The listing builds one solid part. Answer for the finished solid, in the listing's coordinates (mm). A direction names the side the tool comes from. Round coordinates to 2 decimals unless told otherwise and drop trailing zeros. Loops run counter-clockwise (first coordinate to the right, second up) from the corner with the lowest first, then second, coordinate; pieces in that order, holes last. Notation, with made-up numbers: (42, 3.5) -> (96, 3.5) arc R14 cw to (96, 12.5) -> close; hole circle Ø3 at (-32, -2). An arc over 180 degrees is marked (long way). Write each question's results on one line, items separated by ' | '. Start each with the question number.
(1) Flat-ended cylindrical pins translate along their axes: pin 1 (5 mm diameter, centred on x = 145.5, z = 226.5, fed in from +Y); pin 2 (11 mm diameter, centred on x = 145.5, z = 240.5, fed in from -Y); pin 3 (5 mm diameter, centred on x = 146, y = 13, fed in from +Z). Find the tip coordinate at first contact, or state that the pin passes through.
(2) The part is cut by section D-D (x = 16). Determine the outline of the cut face in (y, z).
(3) Straight lines are drawn through the part: probe 1 along Z at (x, y) = (110.5, -95.5); probe 2 along Y at (x, z) = (116.5, -76); probe 3 along X at (y, z) = (-36.5, 268). For each, find the intervals that lie inside material, in ascending order.
(4) Determine the mould class of faces 3 (the face through (-134.971, 135.695, 74.315)), 4 (the face through (144.16, 1.92, 345.07)), 5 (the face through (144, 1, 187.809)) for opening direction Y: released by +Y, released by -Y, zero draft, split by the parting line, or undercut.
(5) The part is cut by section B-B (y = 59.5). Determine the outline of the cut face in (x, z), plus the area to 3 significant figures.
(6) The part is cut by section C-C (z = 55). Determine the outline of the cut face in (x, y), plus the area to 3 significant figures.
(7) The part is cut by section A-A (x = 58). Determine the outline of the cut face in (y, z).
(8) For faces 1 (the face through (-134.971, -134.794, 80.685)), 2 (the face through (88, -95.828, 27)), determine the directions among +Z, -Z, +X, -X, +Y, -Y from which every point of the face is accessible in a straight line to the end or side of a thin tool.
Autodesk Fusion 360 part; units mm, degrees
sketch "Sketch1" plane through (0, 0, 0) normal (0, 0, 1) x (1, 0, 0)
ref_plane "WorkPlane1" through (0, 0, 350) normal (0, 0, 1) x (1, 0, 0)
sketch "Sketch2" plane through (0, 0, 350) normal (0, 0, 1) x (1, 0, 0)
  line L0 (-149.2293, 150.7302) -> (149.2293, 150.7302)
  line L1 (149.2293, 150.7302) -> (149.2293, -149.8296)
  line L2 (149.2293, -149.8296) -> (-149.2293, -149.8296)
  line L3 (-149.2293, -149.8296) -> (-149.2293, 150.7302)
  dimension "d12" = 298.4585
extrude "Extrude1" add sketch "Sketch2" against normal blind 500
fillet "Fillet1" radius 45 2 edges at (0, -149.8296, 350) (0, 150.7302, 350)
sketch "Sketch3" plane through (149.2293, 0, 0) normal (1, 0, 0) x (0, 1, 0)
  arc A0 (150.7302, 305) -> (105.7302, 350) centre (105.7302, 305) ccw
  line L0 (105.7302, 350) -> (-104.8296, 350)
  arc A1 (-104.8296, 350) -> (-149.8296, 305) centre (-104.8296, 305) ccw
  line L1 (-149.8296, 305) -> (-149.8296, -150)
  line L2 (-149.8296, -150) -> (150.7302, -150)
  line L3 (150.7302, -150) -> (150.7302, 305)
  line L4 (-95.4736, 302.4093) -> (94.5264, 302.4093)
  line L5 (94.5264, 302.4093) -> (94.5264, 187.809)
  line L6 (94.5264, 187.809) -> (-95.4736, 187.809)
  line L7 (-95.4736, 187.809) -> (-95.4736, 302.4093)
extrude "Extrude2" cut sketch "Sketch3" against normal blind 10 contours L4 L5 L6 L7
sketch "Sketch4" plane through (149.2293, 0, 0) normal (1, 0, 0) x (0, 1, 0)
  line L0 (94.5264, 302.4093) -> (94.5264, 187.809)
  line L1 (94.5264, 187.809) -> (-95.4736, 187.809)
  line L2 (-95.4736, 187.809) -> (-95.4736, 302.4093)
  line L3 (-95.4736, 302.4093) -> (94.5264, 302.4093)
  arc A0 (150.7302, 305) -> (105.7302, 350) centre (105.7302, 305) ccw
  line L4 (105.7302, 350) -> (-104.8296, 350)
  arc A1 (-104.8296, 350) -> (-149.8296, 305) centre (-104.8296, 305) ccw
  line L5 (-149.8296, 305) -> (-149.8296, -150)
  line L6 (-149.8296, -150) -> (150.7302, -150)
  line L7 (150.7302, -150) -> (150.7302, 305)
  line L8 (-95.828, 164.9511) -> (97.4581, 164.9511)
  line L9 (97.4581, 164.9511) -> (97.4581, -106.9169)
  line L10 (97.4581, -106.9169) -> (-95.828, -106.9169)
  line L11 (-95.828, -106.9169) -> (-95.828, 164.9511)
extrude "Extrude3" cut sketch "Sketch4" against normal blind 150 contours L8 L9 L10 L11
fillet "Fillet2" radius 25 2 edges at (-0.7707, 97.4581, 29.0171) (-0.7707, -95.828, 29.0171)
chamfer "Chamfer1" distance 10 angle 45 5 edges at (149.2293, 150.7302, 77.5) (149.2293, 137.55, 336.8198) (149.2293, 0.4503, 350) (149.2293, -136.6494, 336.8198) (149.2293, -149.8296, 77.5)
fillet "Fillet3" radius 50 5 edges at (-149.2293, 150.7302, 77.5) (-149.2293, 137.55, 336.8198) (-149.2293, 0.4503, 350) (-149.2293, -136.6494, 336.8198) (-149.2293, -149.8296, 77.5)
Checked values:
1) pin 1: stops at y = 146.96 | pin 2: stops at y = -149.06 | pin 3: stops at z = 345.73
2) outline: (-149.83, -150) -> (150.73, -150) -> (150.73, 305) arc R45 ccw to (105.73, 350) -> (-104.83, 350) arc R45 ccw to (-149.83, 305) -> close; hole (-94.43, -106.92) -> (96.06, -106.92) -> (96.06, 164.95) -> (-94.43, 164.95) -> close
3) probe 1: z = -150 to -106.92, 164.95 to 350 | probe 2: y = -149.83 to -95.83, 97.46 to 150.73 | probe 3: x = -149.23 to 139.23
4) face 3: released by +Y | face 4: zero draft | face 5: undercut
5) outline: (-149.23, -150) -> (149.23, -150) -> (149.23, -106.92) -> (-0.77, -106.92) -> (-0.77, 164.95) -> (149.23, 164.95) -> (149.23, 187.81) -> (139.23, 187.81) -> (139.23, 302.41) -> (149.23, 302.41) -> (149.23, 340) -> (139.23, 350) -> (-99.23, 350) arc R50 ccw to (-149.23, 300) -> close | area: 107,000 mm2
6) outline: (-149.23, -99.83) arc R50 ccw to (-99.23, -149.83) -> (139.23, -149.83) -> (149.23, -139.83) -> (149.23, -95.83) -> (24.23, -95.83) arc R25 cw to (-0.77, -70.83) -> (-0.77, 72.46) arc R25 cw to (24.23, 97.46) -> (149.23, 97.46) -> (149.23, 140.73) -> (139.23, 150.73) -> (-99.23, 150.73) arc R50 ccw to (-149.23, 100.73) -> close | area: 59,800 mm2
7) outline: (-149.83, -150) -> (150.73, -150) -> (150.73, 305) arc R45 ccw to (105.73, 350) -> (-104.83, 350) arc R45 ccw to (-149.83, 305) -> close; hole (-95.83, -106.92) -> (97.46, -106.92) -> (97.46, 164.95) -> (-95.83, 164.95) -> close
8) face 1: +Z, -Z, -X, -Y | face 2: +X
